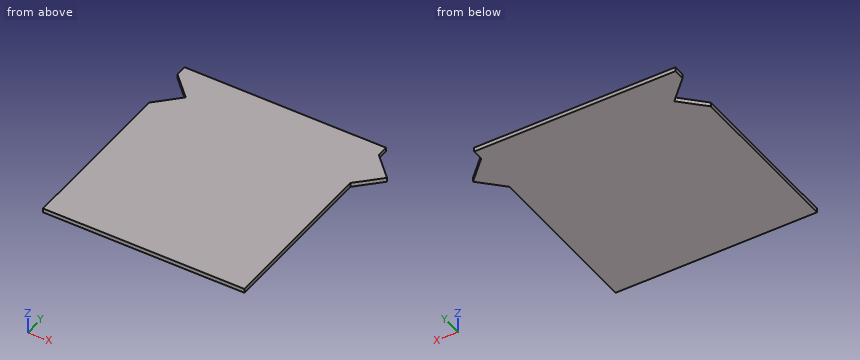
Autodesk Inventor part; units mm, degrees
ref_plane "YZ Plane" through (0, 0, 0) normal (1, 0, 0) x (0, 1, 0)
ref_plane "XZ Plane" through (0, 0, 0) normal (0, 1, 0) x (-1, 0, 0)
ref_plane "XY Plane" through (0, 0, 0) normal (0, 0, 1) x (1, 0, 0)
sketch "Sketch1" plane through (0, 0, 0) normal (0, 0, 1) x (1, 0, 0)
  line L0 (0, 0) -> (-72, 0)
  circle A0 centre (-72, 68) radius 8 construction
  line L1 (-72, 60) -> (0, 60) construction
  line L2 (-72, 76) -> (-64, 68)
  line L3 (-72, 60) -> (-64, 68)
  line L4 (0, 60) -> (0, 0)
  line L5 (-72, 0) -> (-72, 60)
  line L6 (-72, 76) -> (-72, 80)
  line L7 (0, 76) -> (0, 80)
  line L8 (-72, 80) -> (0, 80)
  line L9 (-72, 76) -> (11.0791, 76) construction
  line L10 (-64, 68) -> (11.3495, 68) construction
  line L11 (-72, 60) -> (22.6598, 60) construction
  circle A1 centre (0, 68) radius 8 construction
  line L12 (0, 60) -> (8, 68)
  line L13 (8, 68) -> (0, 76)
  point P0 (0, 0)
  point P1 (0, 78)
  point P2 (-72, 78)
  dimension "d0" = 80
  dimension "d2" = 60
  dimension "d3" = 0
  dimension "d4" = 0
  dimension "d5" = 72
extrude "Extrusion1" add sketch "Sketch1" along normal blind 1.5
properties part number "MS_RI_back_v3"
Source: CAD feature listing. Evaluate the final solid. Frame: model axes, mm. Round coordinates to 2 decimals unless told otherwise and drop trailing zeros. Loops run counter-clockwise (first coordinate to the right, second up) from the corner with the lowest first, then second, coordinate; pieces in that order, holes last. Notation, with made-up numbers: M 52.25,-3 L 62.25,-3 A24 cw 62.25,19 Z; hole C -15.75,18 d2. An arc over 180 degrees is marked long. Use a Markdown table: item, result. Add a question column.
1. Section query A-A on z = 1.2. Return the cut outline in (x, y), then the cut area to 3 significant figures.
2. Section query C-C on y = 66.5. Return the cut outline in (x, z).
3. Line query: line 1 (X direction, y = 47.5, z = 0.5); line 2 (Y direction, x = -65.5, z = 0.25); line 3 (Y direction, x = -65, z = 0.95). Output: solid intervals per line, ascending.
4. Section query B-B on x = 2. Return the cut outline in (y, z).
Reported:
| question | item | result |
|---|---|---|
| 1 | outline | M -72,0 L 0,0 L 0,60 L 8,68 L 0,76 L 0,80 L -72,80 L -72,76 L -64,68 L -72,60 Z |
| 1 | area | 5,760 mm² |
| 2 | outline | M -65.5,0 L 6.5,0 L 6.5,1.5 L -65.5,1.5 Z |
| 3 | line 1 | x = -72 to 0 |
| 3 | line 2 | y = 0 to 66.5, 69.5 to 80 |
| 3 | line 3 | y = 0 to 67, 69 to 80 |
| 4 | outline | M 62,0 L 74,0 L 74,1.5 L 62,1.5 Z |
